Source: three-view drawing plus pictorial views. Frame: mm from the lowest corner of the part. A direction names the side the tool comes from. Round coordinates to 2 decimals unless told otherwise and drop trailing zeros. Write each loop counter-clockwise with the first axis right and the second up, starting at its lowest first coordinate (ties: lowest second). Pieces come first, ordered by that corner, then holes. Notation, with made-up numbers: M -29,56 L -21,56 A25 cw -21,83 Z; hole C 73.25,20 d2. An arc over 180 degrees is marked long. Answer as CSV lines item,"result". Start each with the question number.
Q1. Section query B-B on x = 10. Output: boundary loops of the cut face in (y, z), and give its area (3 significant figures).
Q2. First-contact query: pin 1 (1 mm diameter, centred on x = 9, y = 4, fed in from +Z); pin 2 (5 mm diameter, centred on x = 14.5, y = 12.5, fed in from -Z); pin 3 (3 mm diameter, centred on y = 17.5, z = 15, fed in from +X). Flat tips, straight axial feed; report the tip coordinate or a pass-through.
Q3. Reachability of the marked faces 1 and 2 from +Z, -Z, +X, -X, +Y, -Y: full face, straight path, thin tool, end or side. Return the list, or none.
Q4. Mould query, pull axis X, two halves, no side actions, for the marked faces 3, 4, 5 and 6. Classes: pulls with the +X half, pulls with the -X half, needs draft (parallel to the pull), parting line crosses it, or undercut.
Q5. Section query D-D on x = 16.25. Output: boundary loops of the cut face in (y, z), and give its area (3 significant figures).
Q6. Ray query, probe 1 along Y at (x, z) = (10, 28.3); probe 2 along Z at (x, y) = (14.5, 23.75); probe 3 along X at (y, z) = (21.5, 25.75). Return the intervals inside material, ascending.
Q7. Section query A-A on y = 5. Output: boundary loops of the cut face in (x, z).
Q8. Section query C-C on y = 8.5. Output: boundary loops of the cut face in (x, z), and give its area (3 significant figures).
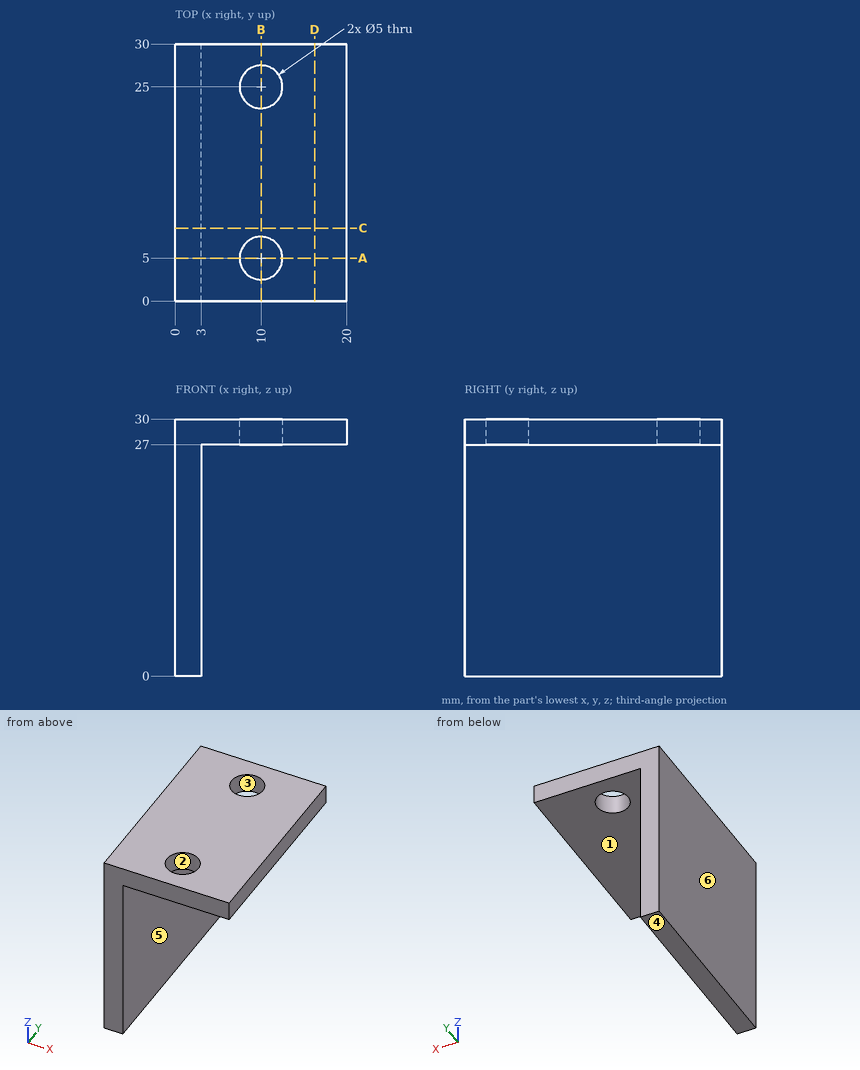
Entries:
1,outline,"M 0,27 L 2.5,27 L 2.5,30 L 0,30 Z; M 7.5,27 L 22.5,27 L 22.5,30 L 7.5,30 Z; M 27.5,27 L 30,27 L 30,30 L 27.5,30 Z"
1,area,"60.0 mm^2"
2,pin 1,"passes through"
2,pin 2,"stops at z = 27"
2,pin 3,"stops at x = 3"
3,face 1,"-Z, +X, +Y, -Y"
3,face 2,"+Z, -Z"
4,face 3,"undercut"
4,face 4,"needs draft"
4,face 5,"pulls with the +X half"
4,face 6,"pulls with the -X half"
5,outline,"M 0,27 L 30,27 L 30,30 L 0,30 Z"
5,area,"90.0 mm^2"
6,probe 1,"y = 0 to 2.5, 7.5 to 22.5, 27.5 to 30"
6,probe 2,"z = 27 to 30"
6,probe 3,"x = 0 to 3"
7,outline,"M 0,0 L 3,0 L 3,27 L 7.5,27 L 7.5,30 L 0,30 Z; M 12.5,27 L 20,27 L 20,30 L 12.5,30 Z"
8,outline,"M 0,0 L 3,0 L 3,27 L 20,27 L 20,30 L 0,30 Z"
8,area,"141 mm^2"
